Work out the finished part from the listing and answer in its coordinate system (mm). A direction names the side the tool comes from. Coordinates: 2 decimals unless noted, no trailing zeros. Loops run counter-clockwise (first coordinate to the right, second up) from the corner with the lowest first, then second, coordinate; pieces in that order, holes last. Notation, with made-up numbers: M -33,66.5 L 9,66.5 A29 ccw 9,100.5 Z; hole C -15.5,42 d11. An arc over 180 degrees is marked long. Write each question's results on one line, items separated by ' | '.
```python
from build123d import *

# Parameters (mm, degrees)
SKETCH042_W             = 102
SKETCH042_H             = 175
PAD011_DEPTH            = 7
SKETCH043_R             = 1.75
POCKET027_DEPTH         = 7.001
SKETCH044_R             = 2.25
POCKET028_DEPTH         = 5
SKETCH045_R             = 2.25
POCKET029_DEPTH         = 5
SKETCH046_W             = 88
SKETCH046_H             = 61
SKETCH046_H_2           = 75.5
POCKET030_DEPTH         = 4
SKETCH047_W             = 186.33641
SKETCH047_H             = 47.448593
POCKET031_DEPTH         = 7.001
BODY010_PLACEMENT_ANGLE = 180


with BuildPart() as part:
    # Sketch042 → Pad011 (new body)
    with BuildSketch(Plane.XY):
        with Locations((51, 87.5)):
            Rectangle(SKETCH042_W, SKETCH042_H)
    extrude(amount=PAD011_DEPTH)

    # Sketch043 (on Face5 of Pad011) → Pocket027 (cut, through all)
    with BuildSketch(Plane(origin=(0, 0, 0), x_dir=(1, 0, 0), z_dir=(0, 0, -1))):
        with Locations((90.6, -129.5)):
            Circle(SKETCH043_R)
        with Locations((14, -129.5)):
            Circle(SKETCH043_R)
        with Locations((90.6, -111.5)):
            Circle(SKETCH043_R)
        with Locations((14, -111.5)):
            Circle(SKETCH043_R)
        with Locations((90.6, -93.5)):
            Circle(SKETCH043_R)
        with Locations((14, -93.5)):
            Circle(SKETCH043_R)
        with Locations((14, -75.5)):
            Circle(SKETCH043_R)
        with Locations((90.6, -75.5)):
            Circle(SKETCH043_R)
        with Locations((90.6, -57.5)):
            Circle(SKETCH043_R)
        with Locations((90.6, -39.5)):
            Circle(SKETCH043_R)
        with Locations((14, -39.5)):
            Circle(SKETCH043_R)
        with Locations((14, -21.5)):
            Circle(SKETCH043_R)
        with Locations((90.6, -21.5)):
            Circle(SKETCH043_R)
        with Locations((14, -57.5)):
            Circle(SKETCH043_R)
    extrude(amount=-POCKET027_DEPTH, mode=Mode.SUBTRACT)

    # Sketch044 (on Face1 of Pocket027) → Pocket028 (cut)
    with BuildSketch(Plane(origin=(0, 0, 0), x_dir=(0, -1, 0), z_dir=(-1, 0, 0))):
        with Locations((-14.5, 3)):
            Circle(SKETCH044_R)
        with Locations((-86.5, 3)):
            Circle(SKETCH044_R)
        with Locations((-140.5, 3)):
            Circle(SKETCH044_R)
    extrude(amount=-POCKET028_DEPTH, mode=Mode.SUBTRACT)

    # Sketch045 (on Face9 of Pocket028) → Pocket029 (cut)
    with BuildSketch(Plane.YZ.offset(102)):
        with Locations((14.5, 3)):
            Circle(SKETCH045_R)
        with Locations((86.5, 3)):
            Circle(SKETCH045_R)
        with Locations((140.5, 3)):
            Circle(SKETCH045_R)
    extrude(amount=-POCKET029_DEPTH, mode=Mode.SUBTRACT)

    # Sketch046 (on Face4 of Pocket029) → Pocket030 (cut)
    with BuildSketch(Plane.XY.offset(7)):
        with Locations((51, 120)):
            Rectangle(SKETCH046_W, SKETCH046_H)
        with Locations((51, 44.75)):
            Rectangle(SKETCH046_W, SKETCH046_H_2)
    extrude(amount=-POCKET030_DEPTH, mode=Mode.SUBTRACT)

    # Sketch047 (on Face4 of Pocket030) → Pocket031 (cut, through all)
    with BuildSketch(Plane.XY.offset(7)):
        with Locations((50.088417, 181.224296)):
            Rectangle(SKETCH047_W, SKETCH047_H)
    extrude(amount=-POCKET031_DEPTH, mode=Mode.SUBTRACT)


with BuildPart() as part_1:
    # Body010 placement: moved
    add(part.part.moved(Location((102, 0, 7))).rotate(Axis((102, 0, 7), (0, 1, 0)), BODY010_PLACEMENT_ANGLE))


solid = part_1.part
```
1) Find section C-C, the plane x = 23. Give the vertices of the cut face in (y, z).
Check result:
outline: M 0,0 L 7,0 L 7,4 L 82.5,4 L 82.5,0 L 89.5,0 L 89.5,4 L 150.5,4 L 150.5,0 L 157.5,0 L 157.5,7 L 0,7 Z
2) Find section A-A, the plane y = 111.5. Give the vertices of the cut face in (x, z), and give its area (3 significant figures).
Check result:
outline: M 0,0 L 7,0 L 7,4 L 9.65,4 L 9.65,7 L 0,7 Z; M 13.15,4 L 86.25,4 L 86.25,7 L 13.15,7 Z; M 89.75,4 L 95,4 L 95,0 L 102,0 L 102,7 L 89.75,7 Z | area: 341 mm^2
3) Straight lines are drawn through the part: probe 1 along X at (y, z) = (39.5, 6.05); probe 2 along Y at (x, z) = (99.25, 4); probe 3 along Y at (x, z) = (19.5, 0.75). For each, find the intervals that lie inside material, in ascending order. Write a range as [from, to].
Check result:
probe 1: [0, 9.65], [13.15, 86.25], [89.75, 102] | probe 2: [0, 12.25], [16.75, 84.25], [88.75, 138.25], [142.75, 157.5] | probe 3: [0, 7], [82.5, 89.5], [150.5, 157.5]
4) Find section B-B, the plane y = 133. Give the vertices of the cut face in (x, z).
Check result:
outline: M 0,0 L 7,0 L 7,4 L 95,4 L 95,0 L 102,0 L 102,7 L 0,7 Z
5) For a pull along Z with two mould halves and no side action, classify faces 5 (the face through (99.54, 12.42, 4.86)), 6 (the face through (52, 45, 4)), 7 (the face through (2.47, 142.58, 4.86)), 8 (the face through (52, 7, 2)) as released by +Z, released by -Z, zero draft, split by the parting line, or undercut.
Check result:
face 5: undercut | face 6: released by -Z | face 7: undercut | face 8: zero draft
6) Find section D-D, the plane x = 88. Give the number of separate pieces and of enclosed holes in the cut face, and give its area (3 significant figures).
Check result:
separate pieces: 8 | enclosed holes: 0 | area: 483 mm^2
7) Which of the six approach directions +Z, -Z, +X, -X, +Y, -Y give full straight-line access (tool end or side, diameter ignored) to faces 1 (the face through (5, 14, 4)), 2 (the face through (97, 141, 4)), 3 (the face through (87.1, 110, 5.5)), 4 (the face through (7, 44, 2))?
Check result:
face 1: -X | face 2: +X | face 3: +Z, -Z | face 4: -Z
8) Given pin 1 Ø12 at (x, y) = (41, 96) entering from -Z; pin 2 Ø3.5 at (y, z) = (14.5, 4) entering from -X; pin 3 Ø2 at (y, z) = (86, 3.5) entering from +X, each flat-ended and moving along its own axis, determine where each tip first touches the part or whether it passes through.
Check result:
pin 1: z = 4 | pin 2: x = 5 | pin 3: x = 97
